from build123d import *

# Parameters (mm, degrees)
F0_R     = 35.5
F1_DEPTH = 6.35
F2_R     = 11
F3_DEPTH = 45.4
F4_R     = 2


with BuildPart() as f1:
    # F0 (on Top) → F1 (new body)
    with BuildSketch(Plane.XY):
        Circle(F0_R)
    extrude(amount=F1_DEPTH)

    # F2 (on face) → F3 (cut)
    with BuildSketch(Plane.XY.offset(6.35)):
        with BuildLine():
            ThreePointArc((-35.4775348505, 1.2627434137), (-17.9359739533, 9.1519318989), (-21.842331384, 27.9850417136))
            ThreePointArc((-21.842331384, 27.9850417136), (-31.6213863215, 16.1349907687), (-35.4775348505, 1.2627434137))
        make_face()
        with BuildLine():
            ThreePointArc((-5.7104578794, 35.0377035607), (-1.8255507227, 35.4530304002), (2.0814687386, 35.4389261673))
            ThreePointArc((2.0814687386, 35.4389261673), (-1.8512627047, 35.9523688566), (-5.7104578794, 35.0377035607))
        make_face()
        with BuildLine():
            ThreePointArc((-5.7104578794, 35.0377035607), (-7.2991901005, 15.7562375394), (9.7144008995, 24.9669228171))
            ThreePointArc((9.7144008995, 24.9669228171), (7.6036569491, 31.4462072594), (2.0814687386, 35.4389261673))
            ThreePointArc((2.0814687386, 35.4389261673), (-1.8255507227, 35.4530304002), (-5.7104578794, 35.0377035607))
        make_face()
        Circle(F2_R)
        with BuildLine():
            ThreePointArc((35.2022114799, 4.58849724), (29.9665998499, 19.032942322), (19.1180348698, 29.9123844372))
            ThreePointArc((19.1180348698, 29.9123844372), (16.9973621306, 10.7956796793), (35.2022114799, 4.58849724))
        make_face()
        with BuildLine():
            ThreePointArc((29.6502759744, -19.5220678884), (32.0612961084, -16.3729438969), (33.1987703135, -12.5734501895))
            ThreePointArc((33.1987703135, -12.5734501895), (31.6160003291, -16.1455418984), (29.6502759744, -19.5220678884))
        make_face()
        with BuildLine():
            ThreePointArc((29.6502759744, -19.5220678884), (31.6160003291, -16.1455418984), (33.1987703135, -12.5734501895))
            ThreePointArc((33.1987703135, -12.5734501895), (33.2482719009, -11.9726798636), (33.2647889641, -11.3700999284))
            ThreePointArc((33.2647889641, -11.3700999284), (12.2089360139, -6.9114205899), (29.6502759744, -19.5220678884))
        make_face()
        with BuildLine():
            ThreePointArc((16.4372598805, -31.465321985), (0.9090375797, -20.1154336224), (-13.5321534944, -32.8196712629))
            ThreePointArc((-13.5321534944, -32.8196712629), (1.6026466455, -35.4638058269), (16.4372598805, -31.465321985))
        make_face()
        with BuildLine():
            ThreePointArc((-27.4883124341, -22.4642533712), (-29.7904496064, -19.3074885019), (-31.731744713, -15.9168582789))
            ThreePointArc((-31.731744713, -15.9168582789), (-30.2100334037, -19.5794249596), (-27.4883124341, -22.4642533712))
        make_face()
        with BuildLine():
            ThreePointArc((-9.9791898636, -13.5968228886), (-22.1457867643, -2.6588591078), (-31.731744713, -15.9168582789))
            ThreePointArc((-31.731744713, -15.9168582789), (-29.7904496064, -19.3074885019), (-27.4883124341, -22.4642533712))
            ThreePointArc((-27.4883124341, -22.4642533712), (-16.009297927, -23.4100881015), (-9.9791898636, -13.5968228886))
        make_face()
    extrude(amount=-F3_DEPTH, mode=Mode.SUBTRACT)

    # F4
    f4_edges = [f1.edges().sort_by_distance(p)[0] for p in [
        (-17.935974, 9.151932, 0),
        (-17.935974, 9.151932, 6.35),
        (16.997362, 10.79568, 0),
        (16.997362, 10.79568, 6.35),
        (0.909038, -20.115434, 0),
        (0.909038, -20.115434, 6.35),
    ]]
    fillet(f4_edges, radius=F4_R)


solid = f1.part
Build history of the part. All positions in model axes, mm. Round coordinates to 2 decimals unless told otherwise and drop trailing zeros. Order: outer loops, then holes, each group sorted by start corner. A loop starts at its lowest first (then second) coordinate and runs counter-clockwise, first axis right, second up. Notation, with made-up numbers: M -13,-35 L 5,-35 A26 ccw 5,-16 Z; hole C 82,21 d3. An arc over 180 degrees is marked long. Use CSV: the item, a comma, the result in double quotes. Start each with the question number.
(1) Cut at A-A on z = 3.5. List the corners of the cut face in (x, y) (1 decimal), then the cut area to 3 significant figures.
(2) Cut at B-B on y = -4. List the corners of the cut face in (x, z), then the cut area to 3 significant figures.
(3) Mould opens along Y. For faces 1 (the face through (35.246, -4.238, 3.131)), 2 (the face through (11.07, 33.73, 3.13)), 3 (the face through (-11, -3, 6.35)), 4 (the face through (16.844, 11.043, 3.191)) say: +Y half, -Y half, draft (parallel to the pull), parting line (faces both ways), or undercut.
(4) Cut at C-C on x = 4.5. State how many separate pieces and enclosed holes the cut face has, then the cut area to 3 significant figures.
(5) Flat gauge pins, fed straight in: P1, Ø8, axis at x = 14, y = 23.5, coming from the +Z side; P2, Ø2, axis at x = -11, z = 0.5, coming from the -Y side; P3, Ø13, axis at x = -1.29, y = 24.97, coming from the +Z side; P4, Ø1, axis at y = 8, z = 2, coming from the -X side. Where does each tip first touch, or does it go through?
(6) Drill centre lines: probe 1 along X at (y, z) = (-6.5, 1.25); probe 2 along X at (y, z) = (-7, 5.5); probe 3 along Y at (x, z) = (-20, 4). Where is each one in solid material? Low to high.
Findings:
1,outline,"M -35.5,1.3 A35.5 ccw -31.7,-15.9 A11 cw long -27.5,-22.5 A35.5 ccw -13.5,-32.8 A15.4 cw 16.4,-31.5 A35.5 ccw 29.7,-19.5 A11 cw long 33.2,-12.6 A35.5 ccw 35.2,4.6 A15.4 cw 19.1,29.9 A35.5 ccw 2.1,35.4 A11 cw long -5.7,35 A35.5 ccw -21.8,28 A15.4 cw Z; hole C 0,0 d22"
1,area,"1,440 mm^2"
2,outline,"M -35.27,0 L -26.36,0 L -26.36,6.35 L -35.27,6.35 Z; M -15.6,0 L -10.25,0 L -10.25,6.35 L -15.6,6.35 Z; M 10.25,0 L 14.1,0 L 14.1,6.35 L 10.25,6.35 Z; M 30.43,0 L 35.27,0 L 35.27,6.35 L 30.43,6.35 Z"
2,area,"146 mm^2"
3,face 1,"parting line"
3,face 2,"+Y half"
3,face 3,"draft"
3,face 4,"undercut"
4,separate pieces,"3"
4,enclosed holes,"0"
4,area,"105 mm^2"
5,P1,"stops at z = 6.35"
5,P2,"stops at y = -27.53"
5,P3,"passes through"
5,P4,"stops at x = -18.91"
6,probe 1,"x = -34.9 to -29.38, -12.57 to -8.87, 8.87 to 12.4, 32.13 to 34.9"
6,probe 2,"x = -34.8 to -29.78, -12.18 to -8.49, 8.49 to 12.17, 32.36 to 34.8"
6,probe 3,"y = -29.33 to -24.55, -2.64 to 6.09, 26.18 to 29.33"
